from build123d import *

# Parameters (mm, degrees)
SKETCH1_W = 37.875561449
SKETCH1_H = 61.587456953
SKETCH2_W = 307.951090162
SKETCH2_H = 19.0499659


with BuildPart() as part:
    # Model → Revolve2 (revolve)
    with BuildSketch(Plane.XY):
        with BuildLine():
            Line((37.9852936, 43.0586642), (169.3032936, 43.0586642))
            ThreePointArc((169.3032936, 43.0586642), (190.401848402, 40.280985836), (210.062572, 32.1372484))
            Line((210.062572, 32.1372484), (228.979018864, 21.215832711))
            ThreePointArc((228.979018864, 21.215832711), (235.369964452, 18.568616337), (242.228293864, 17.665700111))
            ThreePointArc((242.228293864, 17.665700111), (243.484699194, 17.783691074), (244.697169154, 18.133537926))
            add(Edge.make_bspline(
                [(244.697169154, 18.133537926), (271.417135664, 28.637280911), (296.809134664, 34.644355511)],
                knots=[0, 0, 0, 1, 1, 1], degree=2))
            Line((296.809134664, 34.644355511), (297.879592264, 34.897593511))
            Line((297.879592264, 34.897593511), (296.809134664, 47.344355511))
            add(Edge.make_bspline(
                [(244.697169154, 30.833537926), (271.417135664, 41.337280911), (296.809134664, 47.344355511)],
                knots=[0, 0, 0, 1, 1, 1], degree=2))
            Line((244.697169154, 30.833537926), (242.228293864, 30.365700111))
            ThreePointArc((242.228293864, 30.365700111), (235.369964452, 31.268616337), (228.979018864, 33.915832711))
            Line((228.979018864, 33.915832711), (210.062572, 44.8372484))
            ThreePointArc((210.062572, 44.8372484), (190.401848402, 52.980985836), (169.3032936, 55.7586642))
            Line((169.3032936, 55.7586642), (37.9852936, 55.7586642))
            Line((37.9852936, 55.7586642), (37.9852936, 43.0586642))
        make_face()
    revolve(axis=Axis((0, -3.5841e-05, 0), (1, 6e-09, 0)))

    # Sketch1 → Cut-Revolve1 (revolve, cut)
    with BuildSketch(Plane.XY):
        with Locations((299.848811079, 30.793694284)):
            Rectangle(SKETCH1_W, SKETCH1_H)
    revolve(axis=Axis((280.911030354, -3.4193e-05, 0), (1, 0, 0)), mode=Mode.SUBTRACT)

    # Sketch2 → Cut-Revolve2 (revolve, cut)
    with BuildSketch(Plane.XY):
        with Locations((153.975545081, 9.52498295)):
            Rectangle(SKETCH2_W, SKETCH2_H)
    revolve(axis=Axis((0, 0, 0), (1, 0, 0)), mode=Mode.SUBTRACT)


solid = part.part
The model under review builds one solid part; all positions refer to its coordinate system, in mm. A direction names the side the tool comes from. Give positions to 0.01 mm unless a question says otherwise; leave off trailing zeros. Loops run counter-clockwise (first coordinate to the right, second up) from the corner with the lowest first, then second, coordinate; pieces in that order, holes last. Notation, with made-up numbers: (4.5, 82.25) -> (30.5, 82.25) arc R20 ccw to (30.5, 110.25) -> close; hole circle Ø5 at (59.25, 32). An arc over 180 degrees is marked (long way). Put each result on its own line as item: value. Start each with the question number.
1. For faces 1 (the face through (228, 33, 10)), 2 (the face through (240.5, 18.17, 5.72)), list the 3-axis set-ups (+Z, -Z, +X, -X, +Y, -Y) from which the entire face can be reached by the end or side of a thin tool; tool diameter is ignored.
2. Mouldability with a two-part tool opening along Y and no side actions: class faces 3 (the face through (37.985, 29, -33)), 4 (the face through (104.56, -5.61, 42.69)), 5 (the face through (102.725, -44.248, -33.928)), 6 (the face through (228.061, 20.742, 6.532)) as released by +Y, released by -Y, zero draft, split by the parting line, or undercut.
3. Wall thickness on probe 1 along Z at (x, y) = (239.75, 0); probe 2 along Z at (x, y) = (237.25, 0); probe 3 along Y at (x, z) = (264, -22.5): over which ranges is each line inside the solid? List them lowest first.
4. Clearance check with flat-ended pins moving along their axes: P1, Ø4, axis at x = 196.5, y = -22, coming from the +Z side; P2, Ø6, axis at x = 96, z = 25.5, coming from the -Y side; P3, Ø1.5, axis at x = 185.5, y = -13.5, coming from the +Z side. State where each tip first meets the part, or that it passes through.
5. We need section A-A on x = 225. State the section outline as (y, z) points, then the cut area to 3 significant figures.
Determined:
1. face 1: none
1. face 2: +X, -X
2. face 3: zero draft
2. face 4: undercut
2. face 5: split by the parting line
2. face 6: undercut
3. probe 1: -30.48 to -19.05, 19.05 to 30.48
3. probe 2: -30.84 to -19.05, 19.05 to 30.84
3. probe 3: -30.49 to -11.33, 11.33 to 30.49
4. P1: z = 47.29
4. P2: y = -51.02
4. P3: z = 52.67
5. outline: circle Ø72.43 at (0, 0); hole circle Ø47.03 at (0, 0)
5. area: 2,380 mm^2
